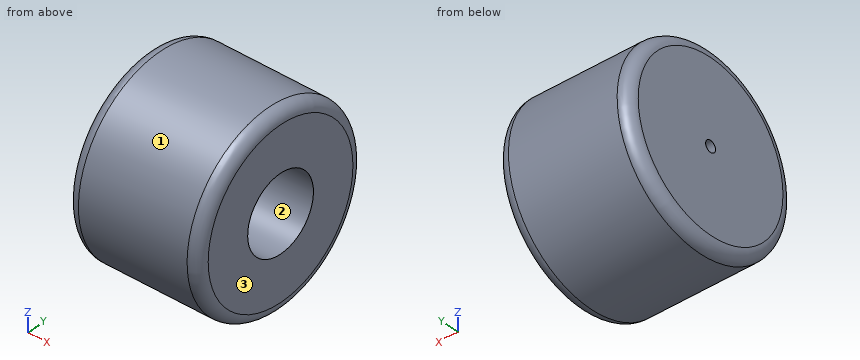
from build123d import *

# Parameters (mm, degrees)
SKETCH1_R           = 25
SKETCH1_R_2         = 1.5
BOSS_EXTRUDE1_DEPTH = 35
SKETCH2_R           = 10
CUT_EXTRUDE1_DEPTH  = 20
FILLET2_R           = 3
FILLET3_R           = 3


with BuildPart() as part:
    # Sketch1 → Boss-Extrude1 (new body)
    with BuildSketch(Plane.YZ):
        with Locations(Location((0, 0, 0), (0, 0, 270))):
            Circle(SKETCH1_R)
        with Locations(Location((0, 0, 0), (0, 0, 270))):
            Circle(SKETCH1_R_2, mode=Mode.SUBTRACT)
    extrude(amount=BOSS_EXTRUDE1_DEPTH)

    # Sketch2 → Cut-Extrude1 (cut)
    with BuildSketch(Plane.YZ.offset(35)):
        with Locations(Location((0, 0, 0), (0, 0, 270))):
            Circle(SKETCH2_R)
    extrude(amount=-CUT_EXTRUDE1_DEPTH, mode=Mode.SUBTRACT)

    # Fillet2
    fillet2_edges = [part.edges().sort_by_distance(p)[0] for p in [
        (0, 0, 25),
    ]]
    fillet(fillet2_edges, radius=FILLET2_R)

    # Fillet3
    fillet3_edges = [part.edges().sort_by_distance(p)[0] for p in [
        (35, 0, 25),
    ]]
    fillet(fillet3_edges, radius=FILLET3_R)


solid = part.part
For this review, take the finished solid that the model builds, in its own axes (mm). Face numbers are marked on the shaded views. Round coordinates to 2 decimals unless told otherwise and drop trailing zeros. Loops run counter-clockwise (first coordinate to the right, second up) from the corner with the lowest first, then second, coordinate; pieces in that order, holes last. Notation, with made-up numbers: (85.25, 11) - (133.25, 11) arc R19 ccw to (133.25, 23) - close; hole circle Ø8 at (32.5, 2.5). An arc over 180 degrees is marked (long way). Use one line per item in the form item = value.
Item 1: Consider section A-A on y = 0. Write out the cut boundary in (x, z), then the cut area to 3 significant figures.
Answers:
outline = (0, -22) arc R3 ccw to (3, -25) - (32, -25) arc R3 ccw to (35, -22) - (35, -10) - (15, -10) - (15, -1.5) - (0, -1.5) - close; (0, 1.5) - (15, 1.5) - (15, 10) - (35, 10) - (35, 22) arc R3 ccw to (32, 25) - (3, 25) arc R3 ccw to (0, 22) - close
area = 1,300 mm^2
Item 2: Clearance check with flat-ended pins moving along their axes: P1, Ø12, axis at x = 7, z = 13, coming from the -Y side; P2, Ø1, axis at y = 0, z = -1.5, coming from the -X side; P3, Ø1, axis at x = 21, y = 11, coming from the +Z side; P4, Ø5, axis at x = 21.5, y = -9, coming from the -Z side. State where each tip first meets the part, or that it passes through.
Answers:
P1 = -24
P2 = 0
P3 = 22.69
P4 = -24.14
Item 3: For line 1 (Y direction, x = 20, z = 0); line 2 (Y direction, x = 6, z = 0); line 3 (Z direction, x = 30, y = -1), list the stretches that pass through material, from the lowest coordinate up.
Answers:
line_1 = -25 to -10, 10 to 25
line_2 = -25 to -1.5, 1.5 to 25
line_3 = -24.98 to -9.95, 9.95 to 24.98
Item 4: Consider section C-C on x = 13.5. Write out the cut boundary in (y, z).
Answers:
outline = circle Ø50 at (0, 0); hole circle Ø3 at (0, 0)
Item 5: Mouldability with a two-part tool opening along Z and no side actions: class the marked faces 1, 2 and 3 as +Z half, -Z half, draft (parallel to the pull), parting line (faces both ways), or undercut.
Answers:
face_1 = parting line
face_2 = undercut
face_3 = draft
